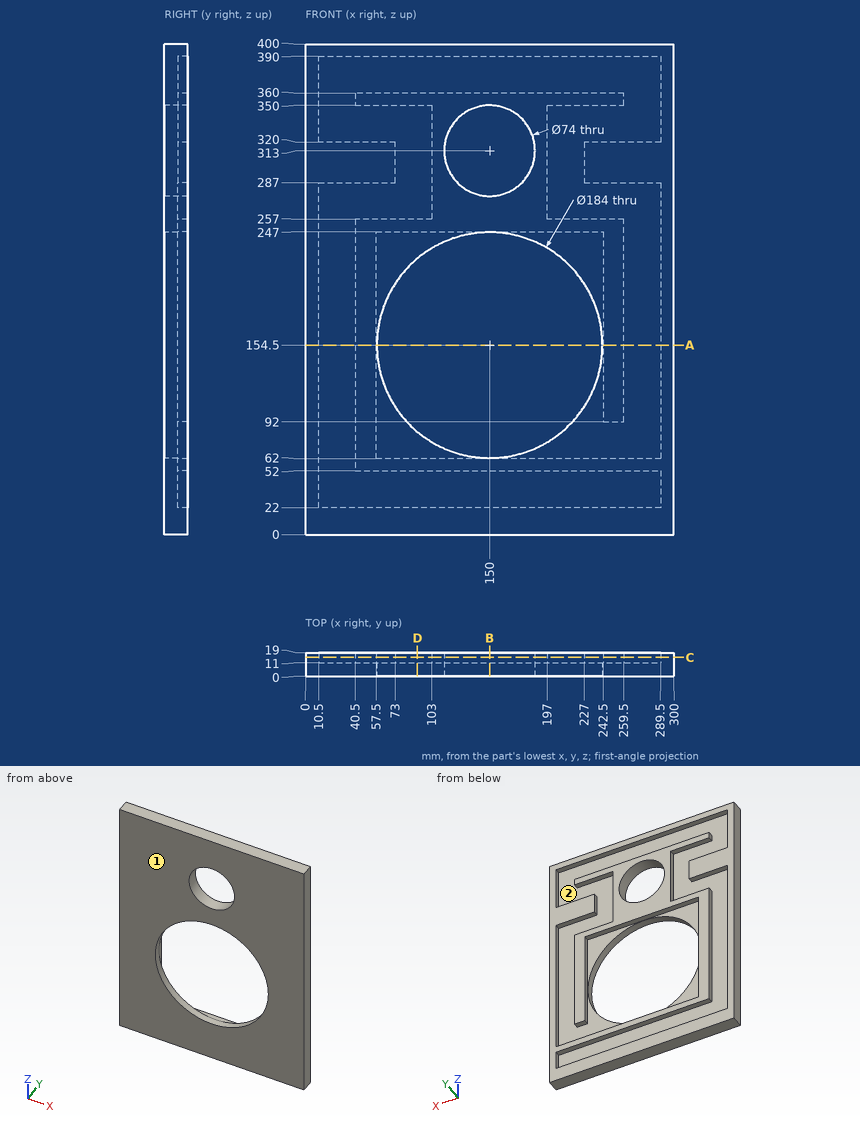
Check sheet for the drawn part. Datum: minimum x, y, z corner. Units: mm. Round coordinates to 2 decimals unless told otherwise and drop trailing zeros. Write each loop counter-clockwise with the first axis right and the second up, starting at its lowest first coordinate (ties: lowest second). Pieces come first, ordered by that corner, then holes. Notation, with made-up numbers: (-15, 5.5) -> (19, 5.5) arc R20 cw to (19, 26.5) -> close; hole circle Ø5 at (86.5, 17.5). An arc over 180 degrees is marked (long way). Write each question's results on one line, items separated by ' | '. Start each with the question number.
1. Material ranges on probe 1 along X at (y, z) = (14.25, 315.5); probe 2 along Z at (x, y) = (102.5, 13.5); probe 3 along Z at (x, y) = (150, 7), recorded low to high. Write a range as from..to.
2. Cross-section at C-C (y = 15.25). Count the separate pieces of the cut face and the enclosed holes in it, then the cut area to 3 significant figures.
3. Cross-section at D-D (x = 91). Enter the section's corners in (y, z).
4. Draft check along Z on the marked faces 1 and 2. Enter one of: +Z half, -Z half, draft (parallel to the pull), parting line (faces both ways), or undercut.
5. Cross-section at A-A (z = 154.5). Enter the section's corners in (x, y).
6. Cross-section at B-B (x = 150). Enter the section's corners in (y, z).
Solutions:
1) probe 1: x = 0..73, 103..113.08, 186.92..197, 227..300 | probe 2: z = 0..22, 52..62, 247..257, 350..360, 390..400 | probe 3: z = 0..62.5, 246.5..276, 350..400
2) separate pieces: 1 | enclosed holes: 2 | area: 38,500 mm2
3) outline: (0, 0) -> (19, 0) -> (19, 22) -> (11, 22) -> (11, 52) -> (19, 52) -> (19, 62) -> (11, 62) -> (11, 83.91) -> (0, 83.91) -> close; (0, 225.09) -> (11, 225.09) -> (11, 247) -> (19, 247) -> (19, 257) -> (11, 257) -> (11, 350) -> (19, 350) -> (19, 360) -> (11, 360) -> (11, 390) -> (19, 390) -> (19, 400) -> (0, 400) -> close
4) face 1: draft | face 2: undercut
5) outline: (0, 0) -> (58, 0) -> (58, 11) -> (57.5, 11) -> (57.5, 19) -> (40.5, 19) -> (40.5, 11) -> (10.5, 11) -> (10.5, 19) -> (0, 19) -> close; (242, 0) -> (300, 0) -> (300, 19) -> (289.5, 19) -> (289.5, 11) -> (259.5, 11) -> (259.5, 19) -> (242.5, 19) -> (242.5, 11) -> (242, 11) -> close
6) outline: (0, 0) -> (19, 0) -> (19, 22) -> (11, 22) -> (11, 52) -> (19, 52) -> (19, 62) -> (11, 62) -> (11, 62.5) -> (0, 62.5) -> close; (0, 246.5) -> (11, 246.5) -> (11, 247) -> (19, 247) -> (19, 276) -> (0, 276) -> close; (0, 350) -> (19, 350) -> (19, 360) -> (11, 360) -> (11, 390) -> (19, 390) -> (19, 400) -> (0, 400) -> close
